Answer from the drawing. Dimensions are ordinates in mm from the lowest x, y and z of the part. Round coordinates to 2 decimals unless told otherwise and drop trailing zeros. Order: outer loops, then holes, each group sorted by start corner. A loop starts at its lowest first (then second) coordinate and runs counter-clockwise, first axis right, second up. Notation, with made-up numbers: M 73.25,-6 L 82.25,-6 A10 ccw 82.25,4 Z; hole C 11,57 d10. An arc over 180 degrees is marked long. Answer as a JSON object with one key per item and string values. Group by question number.
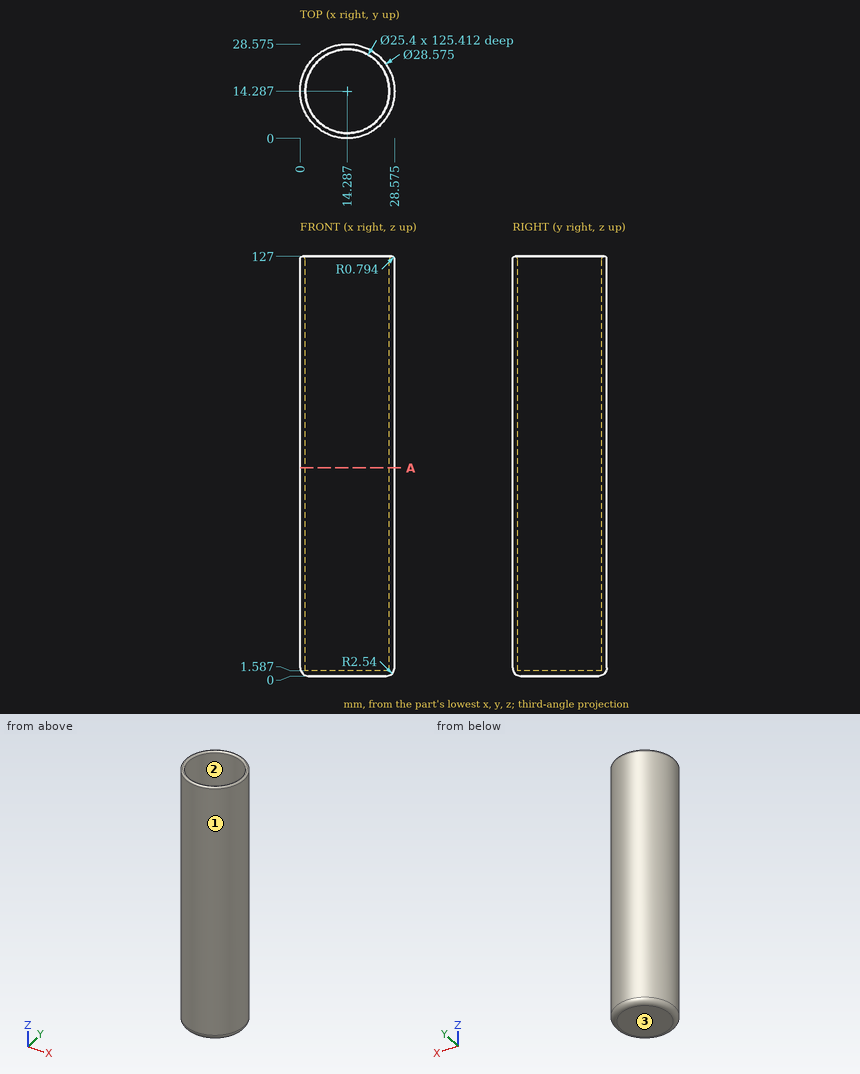
Item 1: Find section A-A (z = 63). Give the vertices of the cut face in (x, y) (1 decimal).
Item 2: The mould has two halves that part along X. Classify the marked faces 1, 2 and 3: +X half, -X half, draft (parallel to the pull), parting line (faces both ways), or undercut.
Item 3: Each of these flat-tipped pins is pushed along its axis until it touches: pin 1 (1 mm diameter, centred on x = 18, y = 3.5, fed in from +Z); pin 2 (5 mm diameter, centred on x = 15, z = 70, fed in from -Y); pin 3 (5 mm diameter, centred on x = 11, z = 58, fed in from +Y); pin 4 (10 mm diameter, centred on x = 20.5, z = 56.5, fed in from +Y). Where does it stop, or does it pass through?
Item 4: Consider L1, parallel to X at y = 13.75, z = 75 (1 decimal); L2, parallel to Y at x = 15, z = 57.5; L3, parallel to X at y = 3.25, z = 48 (1 decimal). Determine where each line is inside the solid, lowest interval first.
Responses:
{
 "1": {"outline": "C 14.3,14.3 d28.6; hole C 14.3,14.3 d25.4"},
 "2": {"face 1": "parting line", "face 2": "undercut", "face 3": "draft"},
 "3": {"pin 1": "stops at z = 1.59", "pin 2": "stops at y = 0", "pin 3": "stops at y = 28.55", "pin 4": "stops at y = 28.52"},
 "4": {"L1": "x = 0 to 1.6, 27 to 28.6", "L2": "y = 0.02 to 1.61, 26.97 to 28.56", "L3": "x = 5.2 to 8, 20.6 to 23.4"}
}
